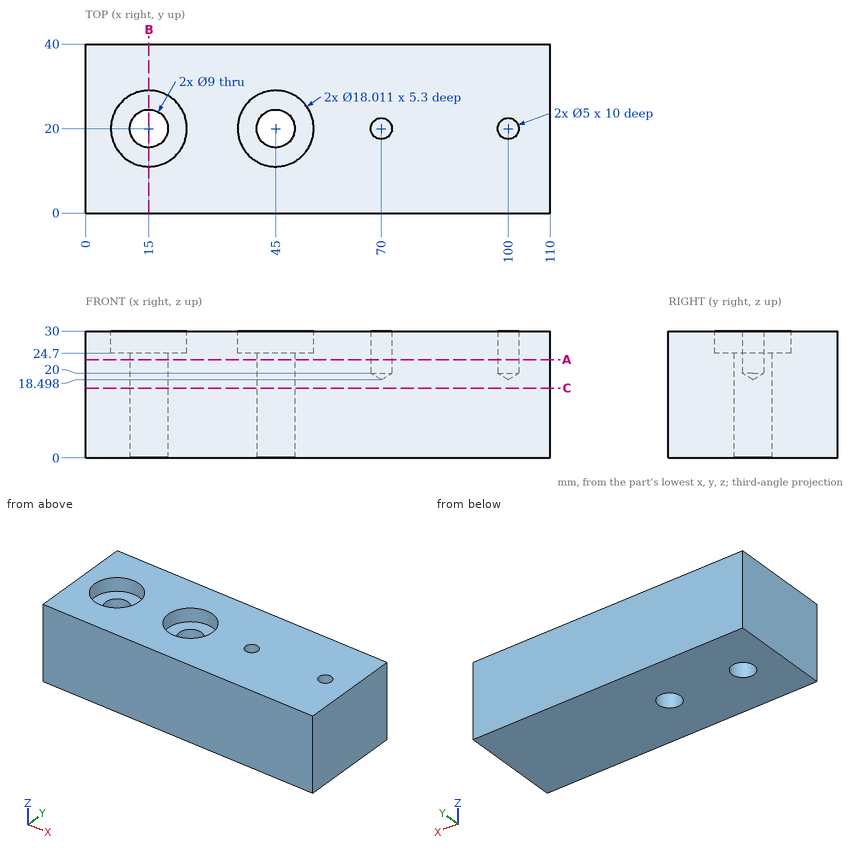
Geometry check sheet. Reference: drawing and pictorial views, mm from the part's lowest x, y, z. Round coordinates to 2 decimals unless told otherwise and drop trailing zeros. Loops run counter-clockwise (first coordinate to the right, second up) from the corner with the lowest first, then second, coordinate; pieces in that order, holes last. Notation, with made-up numbers: (49, 11.5) - (105, 11.5) arc R27 ccw to (105, 48.5) - close; hole circle Ø3 at (-28, -6.5). An arc over 180 degrees is marked (long way). One line per question, with ' | ' between items. Start each with the question number.
1. Scan lines: line 1 (Y direction, x = 45, z = 18.75); line 2 (Y direction, x = 45, z = 28.4); line 3 (X direction, y = 13.5, z = 25.25). Record each from-to range of solid material in increasing order. Write a range as [from, to].
2. Depth check by flat-ended pin: pin 1 (8 mm diameter, centred on y = 25, z = 18, fed in from -X); pin 2 (10.5 mm diameter, centred on x = 15, y = 20, fed in from +Z); pin 3 (4 mm diameter, centred on x = 100, y = 20, fed in from +Z). Enter the tip coordinate at first touch or a pass-through.
3. Cross-section at B-B on x = 15. Record the cut outline in (y, z), then the cut area to 3 significant figures.
4. Cross-section at C-C on z = 16.5. Record the cut outline in (x, y).
5. Cross-section at A-A on z = 23.25. Record the cut outline in (x, y).
Taken from the geometry:
1) line 1: [0, 15.5], [24.5, 40] | line 2: [0, 10.99], [29.01, 40] | line 3: [0, 8.77], [21.23, 38.77], [51.23, 110]
2) pin 1: x = 0 | pin 2: z = 24.7 | pin 3: z = 19.7
3) outline: (0, 0) - (15.5, 0) - (15.5, 24.7) - (10.99, 24.7) - (10.99, 30) - (0, 30) - close; (24.5, 0) - (40, 0) - (40, 30) - (29.01, 30) - (29.01, 24.7) - (24.5, 24.7) - close | area: 882 mm²
4) outline: (0, 0) - (110, 0) - (110, 40) - (0, 40) - close; hole circle Ø9 at (15, 20); hole circle Ø9 at (45, 20)
5) outline: (0, 0) - (110, 0) - (110, 40) - (0, 40) - close; hole circle Ø9 at (15, 20); hole circle Ø9 at (45, 20); hole circle Ø5 at (70, 20); hole circle Ø5 at (100, 20)
